from build123d import *

# Parameters (mm, degrees)
BOSS_EXTRUDE1_DEPTH = 1
SKETCH3_W           = 20
SKETCH3_H           = 87.5
BOSS_EXTRUDE4_DEPTH = 1
CIRPATTERN1_COUNT   = 2
CIRPATTERN1_ANGLE   = 90
CHAMFER1_DEPTH      = 1
SKETCH5_R           = 1.5
BOSS_EXTRUDE6_DEPTH = 1
CHAMFER3_SIZE       = 1


with BuildPart() as part:
    # Sketch1 → Boss-Extrude1 (new body)
    with BuildSketch(Plane(origin=(0, 0, 0), x_dir=(1, 0, 0), z_dir=(0, 1, 0))):
        Polygon((53.75, 5.29391293), (51.684417643, 15.678296686), (47.632632102, 25.460172293), (41.750351221, 34.263627757), (34.263627757, 41.750351221), (25.460172293, 47.632632102), (15.678296686, 51.684417643), (5.29391293, 53.75), (-5.29391293, 53.75), (-15.678296686, 51.684417643), (-25.460172293, 47.632632102), (-34.263627757, 41.750351221), (-41.750351221, 34.263627757), (-47.632632102, 25.460172293), (-51.684417643, 15.678296686), (-53.75, 5.29391293), (-53.75, -5.29391293), (-51.684417643, -15.678296686), (-47.632632102, -25.460172293), (-41.750351221, -34.263627757), (-34.263627757, -41.750351221), (-25.460172293, -47.632632102), (-15.678296686, -51.684417643), (-5.29391293, -53.75), (5.29391293, -53.75), (15.678296686, -51.684417643), (25.460172293, -47.632632102), (34.263627757, -41.750351221), (41.750351221, -34.263627757), (47.632632102, -25.460172293), (51.684417643, -15.678296686), (53.75, -5.29391293), align=None)
        Polygon((43.75, 4.308998897), (42.068712035, 12.76140428), (38.770747059, 20.723396052), (33.982844017, 27.888999337), (27.888999337, 33.982844017), (20.723396052, 38.770747059), (12.76140428, 42.068712035), (4.308998897, 43.75), (-4.308998897, 43.75), (-12.76140428, 42.068712035), (-20.723396052, 38.770747059), (-27.888999337, 33.982844017), (-33.982844017, 27.888999337), (-38.770747059, 20.723396052), (-42.068712035, 12.76140428), (-43.75, 4.308998897), (-43.75, -4.308998897), (-42.068712035, -12.76140428), (-38.770747059, -20.723396052), (-33.982844017, -27.888999337), (-27.888999337, -33.982844017), (-20.723396052, -38.770747059), (-12.76140428, -42.068712035), (-4.308998897, -43.75), (4.308998897, -43.75), (12.76140428, -42.068712035), (20.723396052, -38.770747059), (27.888999337, -33.982844017), (33.982844017, -27.888999337), (38.770747059, -20.723396052), (42.068712035, -12.76140428), (43.75, -4.308998897), align=None, mode=Mode.SUBTRACT)
    extrude(amount=BOSS_EXTRUDE1_DEPTH)

    # Sketch3 → Boss-Extrude4 (add)
    with BuildSketch(Plane(origin=(0, 1, 0), x_dir=(1, 0, 0), z_dir=(0, 1, 0))):
        Rectangle(SKETCH3_W, SKETCH3_H)
    boss_extrude4 = extrude(amount=-BOSS_EXTRUDE4_DEPTH)

    # CirPattern1: Boss-Extrude4 ×2 about axis
    cirpattern1_axis = Axis((0, 1, 0), (0, 1, 0))
    for i in range(1, CIRPATTERN1_COUNT):
        add(boss_extrude4.rotate(cirpattern1_axis, i * CIRPATTERN1_ANGLE / (CIRPATTERN1_COUNT - 1)))

    # Chamfer1: read off the stored shape, not the designer's step
    # Chamfer1 outline → Chamfer1 (add)
    with BuildSketch(Plane(origin=(0, 0, 0), x_dir=(1, 0, 0), z_dir=(0, 1, 0))):
        Polygon((10, -10), (10, -14), (14, -10), align=None)
        Polygon((13.692057296, -41.683222934), (10, -39.216269119), (10, -42.617989498), (12.76140428, -42.068712035), align=None)
        Polygon((42.617989498, -10), (39.216269119, -10), (41.683222934, -13.692057296), (42.068712035, -12.76140428), align=None)
        Polygon((-10, 10), (-10, 14), (-14, 10), align=None)
        Polygon((-13.692057296, 41.683222934), (-10, 39.216269119), (-10, 42.617989498), (-12.76140428, 42.068712035), align=None)
        Polygon((-42.617989498, 10), (-39.216269119, 10), (-41.683222934, 13.692057296), (-42.068712035, 12.76140428), align=None)
        Polygon((10, 10), (14, 10), (10, 14), align=None)
        Polygon((41.683222934, 13.692057296), (39.216269119, 10), (42.617989498, 10), (42.068712035, 12.76140428), align=None)
        Polygon((10, 42.617989498), (10, 39.216269119), (13.692057296, 41.683222934), (12.76140428, 42.068712035), align=None)
        Polygon((-10, -10), (-14, -10), (-10, -14), align=None)
        Polygon((-41.683222934, -13.692057296), (-39.216269119, -10), (-42.617989498, -10), (-42.068712035, -12.76140428), align=None)
        Polygon((-10, -42.617989498), (-10, -39.216269119), (-13.692057296, -41.683222934), (-12.76140428, -42.068712035), align=None)
    extrude(amount=CHAMFER1_DEPTH)

    # Sketch5 → Boss-Extrude6 (add)
    # profile 1 of 3: a face of its own
    with BuildSketch(Plane(origin=(0, 1, 0), x_dir=(1, 0, 0), z_dir=(0, 1, 0))):
        Polygon((-54.729274058, 3.5), (-58.770725942, 3.5), (-60.791451884, 0), (-58.770725942, -3.5), (-54.729274058, -3.5), (-53.75, -3.5), (-53.75, 3.5), align=None)
        with Locations(Location((-56.75, 0, 0), (0, 0, 270))):
            Circle(SKETCH5_R, mode=Mode.SUBTRACT)
    # profile 2 of 3: a face of its own
    with BuildSketch(Plane(origin=(0, 1, 0), x_dir=(1, 0, 0), z_dir=(0, 1, 0))):
        Polygon((54.729274058, 3.5), (53.75, 3.5), (53.75, -3.5), (54.729274058, -3.5), (58.770725942, -3.5), (60.791451884, 0), (58.770725942, 3.5), align=None)
        with Locations(Location((56.75, 0, 0), (0, 0, 270))):
            Circle(SKETCH5_R, mode=Mode.SUBTRACT)
    # profile 3 of 3: a face of its own
    with BuildSketch(Plane(origin=(0, 1, 0), x_dir=(1, 0, 0), z_dir=(0, 1, 0))):
        Polygon((3.5, -54.729274058), (3.5, -53.75), (-3.5, -53.75), (-3.5, -54.729274058), (-3.5, -58.770725942), (0, -60.791451884), (3.5, -58.770725942), align=None)
        with Locations(Location((0, -56.75, 0), (0, 0, 270))):
            Circle(SKETCH5_R, mode=Mode.SUBTRACT)
    extrude(amount=-BOSS_EXTRUDE6_DEPTH)

    # Chamfer3
    chamfer3_edges = [part.edges().sort_by_distance(p)[0] for p in [
        (-53.75, 0.5, 3.5),
        (-53.75, 0.5, -3.5),
        (53.75, 0.5, -3.5),
        (53.75, 0.5, 3.5),
        (3.5, 0.5, 53.75),
        (-3.5, 0.5, 53.75),
    ]]
    chamfer(chamfer3_edges, length=CHAMFER3_SIZE)


solid = part.part
CAD build for the part. Positions are in the model's coordinates, mm. A direction names the side the tool comes from. Coordinates: 2 decimals unless noted, no trailing zeros. Order: outer loops, then holes, each group sorted by start corner. A loop starts at its lowest first (then second) coordinate and runs counter-clockwise, first axis right, second up. Notation, with made-up numbers: (70, -33) -> (125, -33) arc R22 cw to (125, -9) -> close; hole circle Ø8 at (16.25, 23). An arc over 180 degrees is marked (long way). Answer in a Markdown table with one row per item.
1) Flat gauge pins, fed straight in: P1, Ø12, axis at x = -20.5, z = -35.5, coming from the +Y side; P2, Ø0.5, axis at y = 0.5, z = -32, coming from the -X side; P3, Ø0.5, axis at x = 20.5, y = 0.5, coming from the -Z side. Where does each tip first touch, or does it go through?
Check values:
| item | result |
|---|---|
| P1 | y = 1 |
| P2 | x = -43.43 |
| P3 | z = -49.79 |
2) Drill centre lines: line 1 (X direction, y = 0.75, z = 0); line 2 (Z direction, x = -31, y = 0.6); line 3 (X direction, y = 0.45, z = 37). Where is each one in solid material? Low to high.
Check values:
| item | result |
|---|---|
| line 1 | -60.79 to -58.25, -55.25 to 55.25, 58.25 to 60.79 |
| line 2 | -43.93 to -30.87, -10 to 10, 30.87 to 43.93 |
| line 3 | -39.01 to -23.37, -10 to 10, 23.37 to 39.01 |
3) Which spindle directions (+Z, -Z, +X, -X, +Y, -Y) get a long thin tool onto all of the face, cutting with end or side? Do faces 4 (the face through (12, 0.5, -12)), 5 (the face through (-20.501, 0.493, -49.687)). Say none if no direction does.
Check values:
| item | result |
|---|---|
| face 4 | +Y, -Y |
| face 5 | -Z, -X, +Y, -Y |
4) Band-saw the part on C-C (z = 32.5). List the corners of the cut face in (x, y).
Check values:
| item | result |
|---|---|
| outline | (-42.93, 0) -> (-29.37, 0) -> (-29.37, 1) -> (-42.93, 1) -> close; (-10, 0) -> (10, 0) -> (10, 1) -> (-10, 1) -> close; (29.37, 0) -> (42.93, 0) -> (42.93, 1) -> (29.37, 1) -> close |
5) Band-saw the part on B-B (z = 56.75). List the corners of the cut face in (x, y), and give its area (3 significant figures).
Check values:
| item | result |
|---|---|
| outline | (-3.5, 0) -> (-1.5, 0) -> (-1.5, 1) -> (-3.5, 1) -> close; (1.5, 0) -> (3.5, 0) -> (3.5, 1) -> (1.5, 1) -> close |
| area | 4.00 mm2 |
6) Band-saw the part on A-A (x = -56.75). List the corners of the cut face in (y, z).
Check values:
| item | result |
|---|---|
| outline | (0, -3.5) -> (1, -3.5) -> (1, -1.5) -> (0, -1.5) -> close; (0, 1.5) -> (1, 1.5) -> (1, 3.5) -> (0, 3.5) -> close |
7) Mould opens along Z. For faces 1 (the face through (20.64, 0.49, -49.63)), 2 (the face through (44.65, 0.493, 29.924)), 3 (the face through (36.41, 0.49, -24.26)) say: pulls with the +Z half, pulls with the -Z half, needs draft (parallel to the pull), parting line crosses it, or undercut.
Check values:
| item | result |
|---|---|
| face 1 | pulls with the -Z half |
| face 2 | pulls with the +Z half |
| face 3 | undercut |
8) Band-saw the part on D-D (y = 0.35). Give the number of separate pieces and of enclosed holes in the cut face, and give its area (3 significant figures).
Check values:
| item | result |
|---|---|
| separate pieces | 1 |
| enclosed holes | 7 |
| area | 6,340 mm2 |
